Design review of the part built by this model. Coordinates are the model's own, in mm. Face numbers are marked on the shaded views. A direction names the side the tool comes from. Coordinates: 2 decimals unless noted, no trailing zeros. Write each loop counter-clockwise with the first axis right and the second up, starting at its lowest first coordinate (ties: lowest second). Pieces come first, ordered by that corner, then holes.
Q1. Clearance check with flat-ended pins moving along their axes: pin 1 Ø1 at (x, z) = (-14.5, -21.5) entering from -Y; pin 2 Ø4 at (x, y) = (-14.5, 35) entering from -Z; pin 3 Ø10 at (y, z) = (16, 6) entering from +X; pin 4 Ø1 at (x, z) = (-14.5, -9) entering from -Y. State where each tip first meets the part, or that it passes through.
Q2. The part is to be moulded in two halves that separate along Z. For the marked faces 3, 4 and 5, say which applies: +Z half, -Z half, draft (parallel to the pull), parting line (faces both ways), or undercut.
Q3. To check wall thickness, follow probe 1 along Y at (x, z) = (-1.5, 14); probe 2 along X at (y, z) = (11.25, 0); probe 3 along X at (y, z) = (32.5, 0). State the ranges of each line that lie inside material, in increasing order.
Q4. Add section A-A, the plane y = 7. Give the boundary of the cut face in (x, z).
Q5. Machinability: for the marked faces 1 and 2, which of the approach directions +Z, -Z, +X, -X, +Y, -Y give a long, thin tool a straight path to every point of the face, cutting with its end or side? Answer none if there is none.
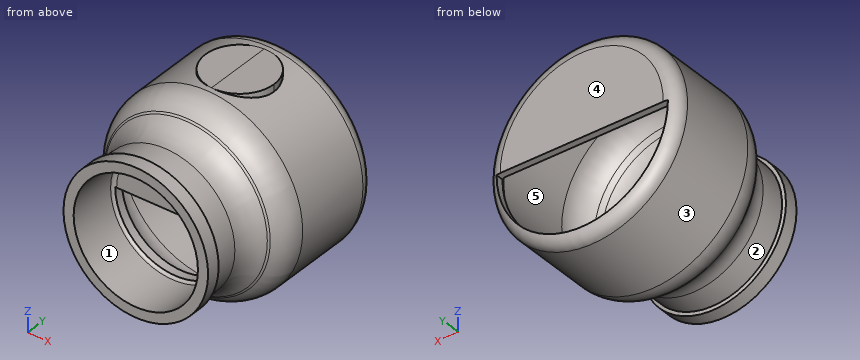
from build123d import *
from build123d.topology import SkipClean

# Parameters (mm, degrees)
CUT_EXTRUDE2_DEPTH      = 25
SKETCH10_R              = 10
BOSS_EXTRUDE1_DEPTH     = 5
CUT_EXTRUDE3_DEPTH      = 5
CUT_EXTRUDE3_DEPTH_BACK = 10


with BuildPart() as part:
    # Sketch1 → Revolve1 (revolve)
    with BuildSketch(Plane.XY):
        with BuildLine():
            Line((20.9, 0), (23.871591838, 0))
            Line((23.871591838, 0), (23.871591838, 4))
            Line((23.871591838, 4), (22.9, 4.236662843))
            Line((22.9, 4.236662843), (22.9, 11.404308102))
            ThreePointArc((22.9, 11.404308102), (23.83692213, 15.63049072), (26.472123903, 19.064752533))
            Line((26.472123903, 19.064752533), (26.988320528, 19.497892931))
            ThreePointArc((26.988320528, 19.497892931), (29.623522302, 22.932154745), (30.560444431, 27.158337362))
            Line((30.560444431, 27.158337362), (30.560444431, 50))
            ThreePointArc((30.560444431, 50), (29.388871556, 52.828427125), (26.560444431, 54))
            Line((26.560444431, 54), (2.764914955, 54))
            Line((2.764914955, 54), (2.764914955, 52))
            Line((2.764914955, 52), (26.560444431, 52))
            ThreePointArc((26.560444431, 52), (27.974657994, 51.414213562), (28.560444431, 50))
            Line((28.560444431, 50), (28.560444431, 28.090952678))
            ThreePointArc((28.560444431, 28.090952678), (27.623522302, 23.864770061), (24.988320528, 20.430508247))
            Line((24.988320528, 20.430508247), (23.688173754, 19.339555569))
            ThreePointArc((23.688173754, 19.339555569), (20.680499091, 17.603073792), (17.260297657, 17))
            Line((17.260297657, 17), (2.764914955, 17))
            Line((2.764914955, 17), (2.764914955, 15))
            Line((2.764914955, 15), (19.9, 15))
            ThreePointArc((19.9, 15), (20.607106781, 14.707106781), (20.9, 14))
            Line((20.9, 14), (20.9, 0))
        make_face()
    revolve(axis=Axis((2.764914955, 7.821821657, 0), (0, 1, 0)))

    # Sketch9 → Cut-Extrude2 (cut)
    with BuildSketch(Plane(origin=(0, 54, 0), x_dir=(1, 0, 0), z_dir=(0, 1, 0))):
        with BuildLine():
            Line((-22.235085045, 0), (27.764914955, 0))
            ThreePointArc((27.764914955, 0), (2.764914955, 25), (-22.235085045, 0))
        make_face()
    extrude(amount=-CUT_EXTRUDE2_DEPTH, mode=Mode.SUBTRACT)

    # Sketch10 → Boss-Extrude1 (add)
    with SkipClean():  # the faces are left unmerged after this step: merging them gives an invalid solid
        with BuildSketch(Plane.XY.offset(27.795529476)):
            with Locations((3.346345887, 38.658337362)):
                Circle(SKETCH10_R)
        extrude(amount=-BOSS_EXTRUDE1_DEPTH)

    # Sketch11 → Cut-Extrude3 (cut, two sides: drawn at the far end of the back side and taken through both)
    with SkipClean():  # the faces are left unmerged after this step: merging them gives an invalid solid
        with BuildSketch(Plane(origin=(0, 17, 0), x_dir=(1, 0, 0), z_dir=(0, 1, 0)).offset(-CUT_EXTRUDE3_DEPTH_BACK)):
            with BuildLine():
                Line((-14.735085045, 0), (20.264914955, 0))
                ThreePointArc((20.264914955, 0), (2.764914955, 17.5), (-14.735085045, 0))
            make_face()
        extrude(amount=CUT_EXTRUDE3_DEPTH + CUT_EXTRUDE3_DEPTH_BACK, mode=Mode.SUBTRACT)


solid = part.part
Here are the results:
1. pin 1: stops at y = 23.43
1. pin 2: stops at z = -23.23
1. pin 3: stops at x = 27.87
1. pin 4: stops at y = 0
2. face 3: parting line
2. face 4: draft
2. face 5: undercut
3. probe 1: y = 15 to 17, 52 to 54
3. probe 2: x = -17.37 to -15.37, 20.9 to 22.9
3. probe 3: x = -25.03 to -23.03, 28.56 to 30.56
4. outline: circle Ø40.27 at (2.76, 0); hole circle Ø36.27 at (2.76, 0)
5. face 1: -Y
5. face 2: none
